from build123d import *

# Parameters (mm, degrees)
SKETCH1_R           = 8.75
BOSS_EXTRUDE1_DEPTH = 1.2
BOSS_EXTRUDE2_DEPTH = 0.5
CIRPATTERN1_COUNT   = 4
SKETCH4_R           = 7.5
BOSS_EXTRUDE3_DEPTH = 1
CUT_EXTRUDE1_REACH  = 96.514
SKETCH6_R           = 1.5
CIRPATTERN2_COUNT   = 4


with BuildPart() as part:
    # Sketch1 → Boss-Extrude1 (new body)
    with BuildSketch(Plane(origin=(0, 0, 0), x_dir=(1, 0, 0), z_dir=(0, 1, 0))):
        with Locations(Location((0, 0, 0), (0, 0, 270))):
            Circle(SKETCH1_R)
    extrude(amount=BOSS_EXTRUDE1_DEPTH)

    # Sketch3 → Boss-Extrude2 (add, symmetric)
    with BuildSketch(Plane(origin=(0, 0, 0), x_dir=(0, 0, -1), z_dir=(1, 0, 0))):
        with BuildLine():
            Line((0, 1.2), (0, 85.2))
            Line((0, 85.2), (6.75, 85.2))
            Line((6.75, 85.2), (6.75, 72.7))
            Line((6.75, 72.7), (3.5, 70.2))
            Line((3.5, 70.2), (6.75, 67.7))
            Line((6.75, 67.7), (6.75, 27.739908728))
            ThreePointArc((6.75, 27.739908728), (6.490167531, 24.69254003), (5.718171558, 21.733149703))
            Line((5.718171558, 21.733149703), (5.531828442, 21.206759025))
            ThreePointArc((5.531828442, 21.206759025), (4.759832469, 18.247368698), (4.5, 15.2))
            Line((4.5, 15.2), (4.5, 1.2))
            Line((4.5, 1.2), (0, 1.2))
        make_face()
    boss_extrude2 = extrude(amount=BOSS_EXTRUDE2_DEPTH, both=True)

    # CirPattern1: Boss-Extrude2 ×4 about axis
    cirpattern1_axis = Axis((0, 0, 0), (0, 1, 0))
    for i in range(1, CIRPATTERN1_COUNT):
        add(boss_extrude2.rotate(cirpattern1_axis, i * 360 / CIRPATTERN1_COUNT))

    # Sketch4 → Boss-Extrude3 (add)
    with BuildSketch(Plane(origin=(0, 85.2, 0), x_dir=(1, 0, 0), z_dir=(0, 1, 0))):
        with Locations(Location((0, 0, 0), (0, 0, 270))):
            Circle(SKETCH4_R)
    extrude(amount=BOSS_EXTRUDE3_DEPTH)

    # Sketch5 → Revolve1 (revolve)
    with BuildSketch(Plane(origin=(0, 0, 0), x_dir=(0, 0, -1), z_dir=(1, 0, 0)), mode=Mode.PRIVATE) as revolve1_sk:
        with BuildLine():
            Line((0, 86.2), (7, 86.2))
            ThreePointArc((7, 86.2), (7.353553391, 86.346446609), (7.5, 86.7))
            Line((7.5, 86.7), (7.5, 90.031561736))
            ThreePointArc((7.5, 90.031561736), (7.331369891, 90.587281183), (6.882351793, 90.955578569))
            Line((6.882351793, 90.955578569), (0.433625988, 93.624016832))
            ThreePointArc((0.433625988, 93.624016832), (0.246188494, 93.680820277), (0.051274196, 93.7))
            Line((0.051274196, 93.7), (0, 93.7))
            Line((0, 93.7), (0, 86.2))
        make_face()
    revolve(revolve1_sk.sketch.rotate(Axis((0, 93.7, 0), (0, -1, 0)), 180), axis=Axis((0, 93.7, 0), (0, -1, 0)))

    # Sketch6 → Cut-Extrude1 (cut, up to next)
    with BuildSketch(Plane.XZ, mode=Mode.PRIVATE) as cut_extrude1_sk1:
        with Locations(Location((3.535533906, -3.535533906, 0), (0, 0, 270))):
            Circle(SKETCH6_R)
    cut_extrude1_tool1 = extrude(cut_extrude1_sk1.sketch, amount=-CUT_EXTRUDE1_REACH, mode=Mode.PRIVATE) & part.part
    cut_extrude1 = cut_extrude1_tool1.solids().sort_by_distance((3.535534, 0, -3.535534))[0]
    add(cut_extrude1, mode=Mode.SUBTRACT)

    # CirPattern2: Cut-Extrude1 ×4 about axis
    cirpattern2_axis = Axis((0, 0, 0), (0, 1, 0))
    for i in range(1, CIRPATTERN2_COUNT):
        add(cut_extrude1.rotate(cirpattern2_axis, i * 360 / CIRPATTERN2_COUNT), mode=Mode.SUBTRACT)


solid = part.part
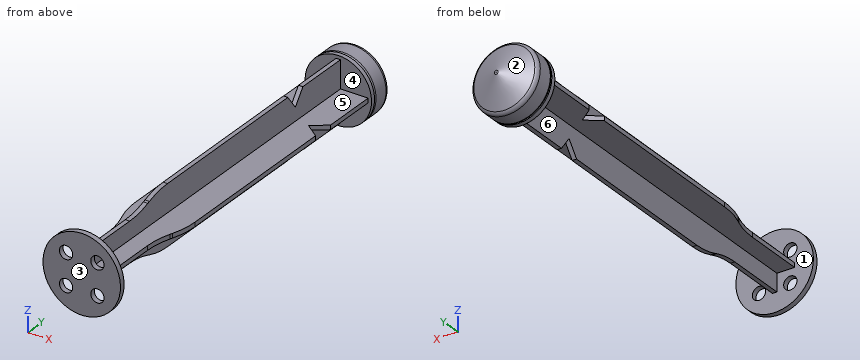
The listing builds one solid part. Answer for the finished solid, in the listing's coordinates (mm). Face numbers are marked on the shaded views. A direction names the side the tool comes from. Give positions to 0.01 mm unless a question says otherwise; leave off trailing zeros. Loops run counter-clockwise (first coordinate to the right, second up) from the corner with the lowest first, then second, coordinate; pieces in that order, holes last. Notation, with made-up numbers: (58, 62.5) - (116, 62.5) arc R7 cw to (116, 66.5) - close; hole circle Ø9 at (37.5, 20). An arc over 180 degrees is marked (long way). Answer as a JSON object with one key per item and string values.
1. Flat-ended cylindrical pins translate along their axes: pin 1 Ø1.1 at (y, z) = (43.5, 0) entering from +X; pin 2 Ø5 at (x, y) = (4, 55.5) entering from -Z; pin 3 Ø0.8 at (y, z) = (9.5, 0) entering from +X. Find the tip coordinate at first contact, or state that the pin passes through.
Determined:
{"pin 1": "x = 6.75", "pin 2": "z = -0.5", "pin 3": "x = 4.5"}
2. Find the intervals of material crossed by L1, parallel to X at y = 51, z = -1.5; L2, parallel to Y at x = -1.25, z = -7.5, in increasing order. Write a range as [from, to].
Determined:
{"L1": "[-0.5, 0.5]", "L2": "[0, 1.2]"}
3. A cutting plane is placed at A-A (y = 10). Write down the section's boundary in (x, z), then the cut area to 3 significant figures.
Determined:
{"outline": "(-4.5, -0.5) - (-0.5, -0.5) - (-0.5, -4.5) - (0.5, -4.5) - (0.5, -0.5) - (4.5, -0.5) - (4.5, 0.5) - (0.5, 0.5) - (0.5, 4.5) - (-0.5, 4.5) - (-0.5, 0.5) - (-4.5, 0.5) - close", "area": "17.0 mm²"}
4. A cutting plane is placed at B-B (y = 23.5). Write down the section's boundary in (x, z), then the cut area to 3 significant figures.
Determined:
{"outline": "(-6.24, -0.5) - (-0.5, -0.5) - (-0.5, -6.24) - (0.5, -6.24) - (0.5, -0.5) - (6.24, -0.5) - (6.24, 0.5) - (0.5, 0.5) - (0.5, 6.24) - (-0.5, 6.24) - (-0.5, 0.5) - (-6.24, 0.5) - close", "area": "24.0 mm²"}
5. For the marked faces 4, 5 and 6, determine the directions among +Z, -Z, +X, -X, +Y, -Y from which every point of the face is accessible in a straight line to the end or side of a thin tool.
Determined:
{"face 4": "none", "face 5": "+Z, +X", "face 6": "-Z, -X"}
6. For a pull along Y with two mould halves and no side action, classify the marked faces 1, 2 and 3 as pulls with the +Y half, pulls with the -Y half, needs draft (parallel to the pull), parting line crosses it, or undercut.
Determined:
{"face 1": "undercut", "face 2": "pulls with the +Y half", "face 3": "pulls with the -Y half"}
